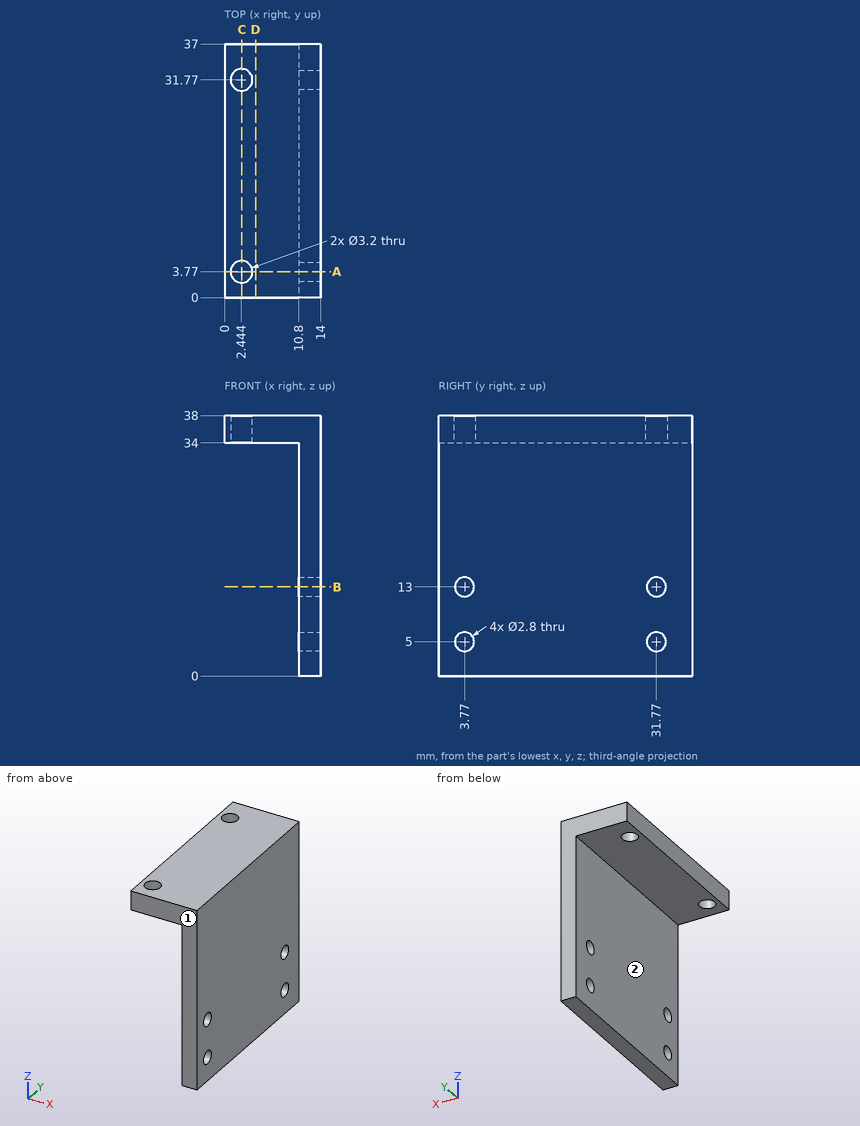
Here's the drawing with two shaded views (mm, measured from the low corner). I have some questions. A direction names the side the tool comes from. Coordinates: 2 decimals unless noted, no trailing zeros. Loops run counter-clockwise (first coordinate to the right, second up) from the corner with the lowest first, then second, coordinate; pieces in that order, holes last. Notation, with made-up numbers: M 16.25,78.5 L 29.25,78.5 A27 ccw 29.25,107.5 Z; hole C 35.25,-0.5 d11. An arc over 180 degrees is marked long. Put each result on its own line as item: value. Start each with the question number.
(1) I need wall thicknesses on probe 1 along Y at (x, z) = (12.8, 13); probe 2 along X at (y, z) = (30.5, 4); probe 3 along Z at (x, y) = (10, 30.5). Which ranges of each line are inside material? Lowest first, please.
(2) Will these pins go through, and if not, where does the flat tip stop? pin 1 Ø2 at (y, z) = (16, 6) entering from -X; pin 2 Ø4 at (x, y) = (2.44, 3.77) entering from -Z.
(3) Imagine slicing it at B-B on z = 13. List the corners of the cut face in (x, y) for me.
(4) Imagine slicing it at D-D on x = 4.5. List the corners of the cut face in (y, z) for me, and give its area (3 significant figures).
(5) Which directions (+Z, -Z, +X, -X, +Y, -Y) give clear straight access to the entire face, cutting with the end or side of a thin tool? Please do the marked faces 1 and 2.
(6) Imagine slicing it at C-C on x = 2.5. List the corners of the cut face in (y, z) for me.
(7) Imagine slicing it at A-A on y = 3.77. List the corners of the cut face in (x, z) for me (1 decimal).
Worked answers:
1. probe 1: y = 0 to 2.37, 5.17 to 30.37, 33.17 to 37
1. probe 2: x = 10.8 to 14
1. probe 3: z = 34 to 38
2. pin 1: stops at x = 10.8
2. pin 2: stops at z = 34
3. outline: M 10.8,0 L 14,0 L 14,2.37 L 10.8,2.37 Z; M 10.8,5.17 L 14,5.17 L 14,30.37 L 10.8,30.37 Z; M 10.8,33.17 L 14,33.17 L 14,37 L 10.8,37 Z
4. outline: M 0,34 L 37,34 L 37,38 L 0,38 Z
4. area: 148 mm2
5. face 1: +Z, -Z, +X, -X, -Y
5. face 2: -Z, -X, +Y, -Y
6. outline: M 0,34 L 2.17,34 L 2.17,38 L 0,38 Z; M 5.37,34 L 30.17,34 L 30.17,38 L 5.37,38 Z; M 33.37,34 L 37,34 L 37,38 L 33.37,38 Z
7. outline: M 0,34 L 0.8,34 L 0.8,38 L 0,38 Z; M 4,34 L 10.8,34 L 10.8,14.4 L 14,14.4 L 14,38 L 4,38 Z; M 10.8,0 L 14,0 L 14,3.6 L 10.8,3.6 Z; M 10.8,6.4 L 14,6.4 L 14,11.6 L 10.8,11.6 Z
